Input: part model. Units: mm. Frame: model coordinates. A direction names the side the tool comes from. Coordinates: 2 decimals unless noted, no trailing zeros. Write each loop counter-clockwise with the first axis right and the second up, starting at its lowest first coordinate (ties: lowest second). Pieces come first, ordered by that corner, then holes.
1) Set-up query: faces 4 (the cylindrical face through (1.36, 7.44, 7.12)), 5 (the conical face through (-0.21, 2.41, 2.92)), 6 (the flat face through (-3, 4, 4)). Return all of +Z, -Z, +X, -X, +Y, -Y with unobstructed straight access to the full face (end or side cutting, diameter ignored); none if empty.
2) Section query B-B (y = 5). Output: boundary loops of the cut face in (x, z).
3) Section query C-C (z = 14.75). Output: boundary loops of the cut face in (x, y), then the cut area to 3 significant figures.
4) Section query A-A (z = 1). Output: boundary loops of the cut face in (x, y).
5) Draft query along X for faces 1 (the cylindrical face through (-1.84, -8.3, 4.44)), 2 (the flat face through (1, -3, 16)), 3 (the flat face through (0, 2.15, 2)). Return one class per face: pulls with the +X half, pulls with the -X half, needs draft (parallel to the pull), parting line crosses it, or undercut.
6) Section query D-D (y = 0). Output: boundary loops of the cut face in (x, z).
7) Line query: L1, parallel to Y at x = 0, z = 8.5; L2, parallel to Z at x = 0, y = 7.25; L3, parallel to Z at x = 7.25, y = 2. Output: solid intervals per line, ascending.
8) Pin query (flat end, axial travel): pin 1 Ø2 at (y, z) = (4, 2.5) entering from -X; pin 2 Ø2 at (y, z) = (-2, 12.5) entering from -X; pin 3 Ø1 at (y, z) = (1, 7.5) entering from +X. Return the tip coordinate at first contact, or that it passes through.
from build123d import *

# Parameters (mm, degrees)
ESQUISSE1_R             = 8.5
BOSS_EXTRU_1_DEPTH      = 9
ESQUISSE2_W             = 6
ESQUISSE2_H             = 2.6
ENL_V_MAT_EXTRU_1_DEPTH = 16.016657418
ESQUISSE7_R             = 2.95
ENL_V_MAT_EXTRU_8_DEPTH = 21.868397324
ESQUISSE9_R             = 3.95
BOSS_EXTRU_2_DEPTH      = 7
ENL_V_MAT_EXTRU_9_DEPTH = 21.012496182


with BuildPart() as part:
    # Esquisse1 → Boss.-Extru.1 (new body)
    with BuildSketch(Plane.XY):
        Circle(ESQUISSE1_R)
    extrude(amount=BOSS_EXTRU_1_DEPTH)

    # Esquisse2 → Enlèv. mat.-Extru.1 (cut, through all)
    with BuildSketch(Plane(origin=(0, 0, 0), x_dir=(-1, 0, 0), z_dir=(0, 0, -1))):
        with Locations((0, 4)):
            Rectangle(ESQUISSE2_W, ESQUISSE2_H)
    extrude(amount=-ENL_V_MAT_EXTRU_1_DEPTH, mode=Mode.SUBTRACT)

    # Enlèv. mat.-Extru.2: read off the stored shape, not the designer's step
    # Enlèv. mat.-Extru.2 outline → Enlèv. mat.-Extru.2 (revolve, cut)
    with BuildSketch(Plane.XY.offset(4.5)):
        Polygon((0, 5.3), (1.554616831, 5.3), (1.498760014, 8.500034923), (0, 8.500034923), align=None)
        Polygon((1.6, 2.7), (0, 2.7), (0, 0.7), (1.56508987, 0.7), align=None)
    revolve(axis=Axis((0, 0, 4.5), (0, 1, 0)), mode=Mode.SUBTRACT)

    # Esquisse7 → Enlèv. mat.-Extru.8 (cut, through all)
    with BuildSketch(Plane(origin=(0, 8.3, 0), x_dir=(1, 0, 0), z_dir=(0, 1, 0))):
        with Locations((0, -4.5)):
            Circle(ESQUISSE7_R)
    extrude(amount=ENL_V_MAT_EXTRU_8_DEPTH, mode=Mode.SUBTRACT)

    # Chanfrein1: read off the stored shape, not the designer's step
    # Chanfrein1 outline → Chanfrein1 (revolve, cut)
    with BuildSketch(Plane.XY.offset(4.5)):
        Polygon((2.95, 6.747748364), (2.95, 8.3), (1.502251636, 8.3), (1.553718474, 5.351466838), align=None)
    revolve(axis=Axis((0, 0, 4.5), (0, 1, 0)), mode=Mode.SUBTRACT)

    # Esquisse9 → Boss.-Extru.2 (add)
    with BuildSketch(Plane.XY.offset(9)):
        with Locations(Location((0, -1, 0), (0, 0, 110.493999506))):
            Circle(ESQUISSE9_R)
    extrude(amount=BOSS_EXTRU_2_DEPTH)

    # Esquisse10 → Enlèv. mat.-Extru.9 (cut, through all)
    with BuildSketch(Plane(origin=(0, 0, 0), x_dir=(-1, 0, 0), z_dir=(0, 0, -1))):
        with BuildLine():
            Line((-1.549193338, 2.15), (1.549193338, 2.15))
            ThreePointArc((1.549193338, 2.15), (0, -2.65), (-1.549193338, 2.15))
        make_face()
    extrude(amount=-ENL_V_MAT_EXTRU_9_DEPTH, mode=Mode.SUBTRACT)


solid = part.part
Answer:
1. face 4: +Y
1. face 5: none
1. face 6: +Z, -Z
2. outline: (-6.87, 0) - (-3, 0) - (-3, 9) - (-6.87, 9) - close; (3, 0) - (6.87, 0) - (6.87, 9) - (3, 9) - close
3. outline: circle Ø7.9 at (0, -1); hole (-1.55, 2.15) arc R2.65 ccw (long way) to (1.55, 2.15) - close
3. area: 28.0 mm2
4. outline: circle Ø17 at (0, 0); hole (-3, 2.7) - (3, 2.7) - (3, 5.3) - (-3, 5.3) - close; hole (-1.55, 2.15) arc R2.65 ccw (long way) to (1.55, 2.15) - close
5. face 1: parting line crosses it
5. face 2: needs draft
5. face 3: undercut
6. outline: (-8.5, 0) - (-2.65, 0) - (-2.65, 16) - (-3.82, 16) - (-3.82, 9) - (-8.5, 9) - close; (2.65, 0) - (8.5, 0) - (8.5, 9) - (3.82, 9) - (3.82, 16) - (2.65, 16) - close
7. L1: y = -8.5 to -2.65, 2.15 to 2.7, 5.3 to 8.5
7. L2: z = 0 to 1.55, 7.45 to 9
7. L3: z = 0 to 9
8. pin 1: stops at x = -7.95
8. pin 2: stops at x = -3.95
8. pin 3: stops at x = 8.49
